```python
from build123d import *

# Parameters (mm, degrees)
SKETCH1_W               = 184
SKETCH1_H               = 15
BOSS_EXTRUDE1_DEPTH     = 7.25
CUT_EXTRUDE1_START      = -7.25
SKETCH1_6_W             = 184
SKETCH1_6_H             = 11
CUT_EXTRUDE1_DEPTH      = 3.5
CUT_EXTRUDE2_DEPTH      = 93.589483744
CUT_EXTRUDE2_DEPTH_BACK = 93.589483744
SKETCH2_R               = 2.25
SKETCH2_R_2             = 1.7
CHAMFER1_SIZE           = 0.4


with BuildPart() as part:
    # Sketch1 → Boss-Extrude1 (new body)
    with BuildSketch(Plane.XY):
        Rectangle(SKETCH1_W, SKETCH1_H)
    extrude(amount=-BOSS_EXTRUDE1_DEPTH)

    # Sketch1<6> → Cut-Extrude1 (cut)
    with BuildSketch(Plane.XY.offset(CUT_EXTRUDE1_START)):
        with Locations((0, -2)):
            Rectangle(SKETCH1_6_W, SKETCH1_6_H)
    extrude(amount=CUT_EXTRUDE1_DEPTH, mode=Mode.SUBTRACT)

    # Sketch2 → Cut-Extrude2 (cut, two sides: drawn at the far end of the back side and taken through both)
    with BuildSketch(Plane.XY.offset(-CUT_EXTRUDE2_DEPTH_BACK)):
        with Locations((-52.5, 0)):
            Circle(SKETCH2_R)
        with Locations((-36.25, 0)):
            Circle(SKETCH2_R_2)
        with Locations((-10.5, 0)):
            Circle(SKETCH2_R)
        Circle(SKETCH2_R_2)
        with Locations((10.5, 0)):
            Circle(SKETCH2_R)
        with Locations((36.25, 0)):
            Circle(SKETCH2_R_2)
        with Locations((52.5, 0)):
            Circle(SKETCH2_R)
    extrude(amount=CUT_EXTRUDE2_DEPTH + CUT_EXTRUDE2_DEPTH_BACK, mode=Mode.SUBTRACT)

    # Chamfer1
    chamfer1_edges = [part.edges().sort_by_distance(p)[0] for p in [
        (-54.75, 0, 0),
        (-37.95, 0, 0),
        (-12.75, 0, 0),
        (-1.7, 0, 0),
        (8.25, 0, 0),
        (34.55, 0, 0),
        (50.25, 0, 0),
        (0, -7.5, 0),
        (-92, 0, 0),
        (0, 7.5, 0),
        (92, 0, 0),
    ]]
    chamfer(chamfer1_edges, length=CHAMFER1_SIZE)


solid = part.part
```
The model under review builds one solid part; all positions refer to its coordinate system, in mm. A direction names the side the tool comes from. Round coordinates to 2 decimals unless told otherwise and drop trailing zeros. Order: outer loops, then holes, each group sorted by start corner. A loop starts at its lowest first (then second) coordinate and runs counter-clockwise, first axis right, second up.
(1) Take a section at C-C, the plane x = -79. State the section outline as (y, z) points, plus the area to 3 significant figures.
Working result:
outline: (-7.5, -3.75) - (3.5, -3.75) - (3.5, -7.25) - (7.5, -7.25) - (7.5, -0.4) - (7.1, 0) - (-7.1, 0) - (-7.5, -0.4) - close
area: 70.1 mm2
(2) Tool access review of faces 4 (the face through (-1, -2, -3.75)), 5 (the face through (-1, -7.5, -2)): name each direction out of +Z, -Z, +X, -X, +Y, -Y from which nothing blocks a thin tool from reaching the whole face with its end or side.
Working result:
face 4: -Z, +X, -X, -Y
face 5: +Z, -Z, +X, -X, -Y
(3) Take a section at B-B, the plane z = -1.75. State the section outline as (x, y) points, plus the area to 3 significant figures.
Working result:
outline: (-92, -7.5) - (92, -7.5) - (92, 7.5) - (-92, 7.5) - close; hole circle Ø4.5 at (-52.5, 0); hole circle Ø3.4 at (-36.25, 0); hole circle Ø4.5 at (-10.5, 0); hole circle Ø3.4 at (0, 0); hole circle Ø4.5 at (10.5, 0); hole circle Ø3.4 at (36.25, 0); hole circle Ø4.5 at (52.5, 0)
area: 2,670 mm2
(4) Take a section at D-D, the plane x = 10.5. State the section outline as (y, z) points, plus the area to 3 significant figures.
Working result:
outline: (-7.5, -3.75) - (-2.25, -3.75) - (-2.25, -0.4) - (-2.65, 0) - (-7.1, 0) - (-7.5, -0.4) - close; (2.25, -3.75) - (3.5, -3.75) - (3.5, -7.25) - (7.5, -7.25) - (7.5, -0.4) - (7.1, 0) - (2.65, 0) - (2.25, -0.4) - close
area: 53.1 mm2
(5) Take a section at A-A, the plane x = 36.25. State the section outline as (y, z) points, plus the area to 3 significant figures.
Working result:
outline: (-7.5, -3.75) - (-1.7, -3.75) - (-1.7, -0.4) - (-2.1, 0) - (-7.1, 0) - (-7.5, -0.4) - close; (1.7, -3.75) - (3.5, -3.75) - (3.5, -7.25) - (7.5, -7.25) - (7.5, -0.4) - (7.1, 0) - (2.1, 0) - (1.7, -0.4) - close
area: 57.2 mm2
(6) Wall thickness on L1, parallel to Y at x = 36.25, z = -1.05; L2, parallel to Y at x = -10.5, z = -2.9; L3, parallel to Z at x = 66.5, y = -4.5: over which ranges is each line inside the solid? List them lowest first.
Working result:
L1: y = -7.5 to -1.7, 1.7 to 7.5
L2: y = -7.5 to -2.25, 2.25 to 7.5
L3: z = -3.75 to 0
(7) For P1, Ø5.5, axis at x = -45.5, y = -0.5, coming from the -Z side, flat-tipped, find the tip position at first contact; note if it passes through.
Working result:
P1: stops at z = -3.75
(8) Mouldability with a two-part tool opening along X and no side actions: class faces 1 (the face through (-1, 3.5, -6)), 2 (the face through (-54.748, 0.099, -2.098)), 3 (the face through (-92, 2, -2)) as released by +X, released by -X, zero draft, split by the parting line, or undercut.
Working result:
face 1: zero draft
face 2: undercut
face 3: released by -X
